Print and shaded views of the part. All mm, measured from the part's lowest x, y and z. Coordinates: 2 decimals unless noted, no trailing zeros. Loops run counter-clockwise (first coordinate to the right, second up) from the corner with the lowest first, then second, coordinate; pieces in that order, holes last. Notation, with made-up numbers: (67, -33.5) -> (122, -33.5) arc R18 cw to (122, -12.5) -> close; hole circle Ø2 at (80.25, 20). An arc over 180 degrees is marked (long way). One line per item, written item: value. Start each with the question number.
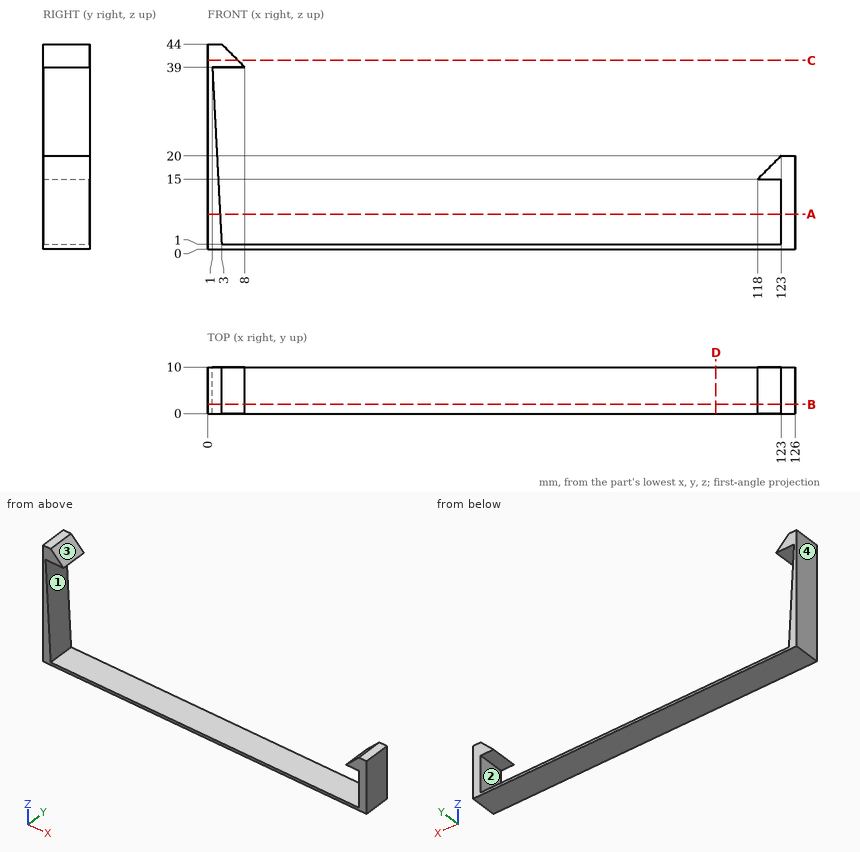
1) Slice it at D-D (x = 109). Give the cut face in (y, z), then the cut area to 3 significant figures.
2) Pull direction Z, two halves, no side cores. Call the marked faces 1, 2, 3 and 4: +Z half, -Z half, draft (parallel to the pull), parting line (faces both ways), or undercut.
3) Probe line 1 (Z direction, x = 90, y = 9); line 2 (Z direction, x = 5.5, y = 6); line 3 (X direction, y = 7.75, z = 18). List the from-to ranges inside material, lowest first. Write a range as from..to.
4) Slice it at A-A (z = 7.5). Give the cut face in (x, y), then the cut area to 3 significant figures.
5) Slice it at B-B (y = 2). Give the cut face in (x, z).
6) Slice it at C-C (z = 40.5). Give the cut face in (x, y), then the cut area to 3 significant figures.
7) Pin check, flat tips, straight feed: pin 1 Ø5 at (y, z) = (1, 29.5) entering from +X; pin 2 Ø1.5 at (x, y) = (124.5, 7) entering from +Z; pin 3 Ø3 at (x, y) = (49.5, 7) entering from +Z. Stop position of each tip, or through.
Check sheet entries:
1. outline: (0, 0) -> (10, 0) -> (10, 1) -> (0, 1) -> close
1. area: 10.0 mm^2
2. face 1: undercut
2. face 2: undercut
2. face 3: +Z half
2. face 4: draft
3. line 1: z = 0..1
3. line 2: z = 0..1, 39..41.5
3. line 3: x = 0..2.11, 121..126
4. outline: (0, 0) -> (2.66, 0) -> (2.66, 10) -> (0, 10) -> close; (123, 0) -> (126, 0) -> (126, 10) -> (123, 10) -> close
4. area: 56.6 mm^2
5. outline: (0, 0) -> (126, 0) -> (126, 20) -> (123, 20) -> (118, 15) -> (123, 15) -> (123, 1) -> (3, 1) -> (1, 39) -> (8, 39) -> (3, 44) -> (0, 44) -> close
6. outline: (0, 0) -> (6.5, 0) -> (6.5, 10) -> (0, 10) -> close
6. area: 65.0 mm^2
7. pin 1: stops at x = 1.63
7. pin 2: stops at z = 20
7. pin 3: stops at z = 1
